The drawing under review shows one solid part. Ordinate dimensions are in mm from its lowest x, y, z. A direction names the side the tool comes from. Coordinates: 2 decimals unless noted, no trailing zeros. Order: outer loops, then holes, each group sorted by start corner. A loop starts at its lowest first (then second) coordinate and runs counter-clockwise, first axis right, second up. Notation, with made-up numbers: (-19.75, -35) -> (-1.75, -35) arc R22 cw to (-1.75, -26) -> close; hole circle Ø11 at (71, 2). An arc over 180 degrees is marked (long way). Use a Markdown table: item, result. Add a question column.
Q1. Add section A-A (x = 13.5). State the section outline as (y, z) points.
Q2. Machinability: for the marked faces 1 and 2, which of the approach directions +Z, -Z, +X, -X, +Y, -Y give a long, thin tool a straight path to every point of the face, cutting with its end or side? Answer none if there is none.
Q3. The part is to be moulded in two halves that separate along Y. For the marked faces 3, 4 and 5, say which applies: pulls with the +Y half, pulls with the -Y half, needs draft (parallel to the pull), parting line crosses it, or undercut.
Q4. Insertion check: pin 1 (0.9 mm diameter, centred on x = 9.5, z = 2.5, fed in from +Y); pin 2 (1.2 mm diameter, centred on y = 8, z = 1, fed in from +X); pin 3 (0.8 mm diameter, centred on y = 44.5, z = 1.5, fed in from +X). Each pin has a flat end and moves straight along its axis. Give the tip position at first contact, or say it passes through.
Q5. Add section B-B (y = 42.5). State the section outline as (x, z) points, then the cut area to 3 significant figures.
Q6. Add section C-C (x = 17). State the section outline as (y, z) points.
Q7. Wall thickness on probe 1 along Y at (x, z) = (11.5, 2); probe 2 along Y at (x, z) = (8.5, 0.7); probe 3 along Y at (x, z) = (14.25, 2.4): over which ranges is each line inside the solid? List them lowest first.
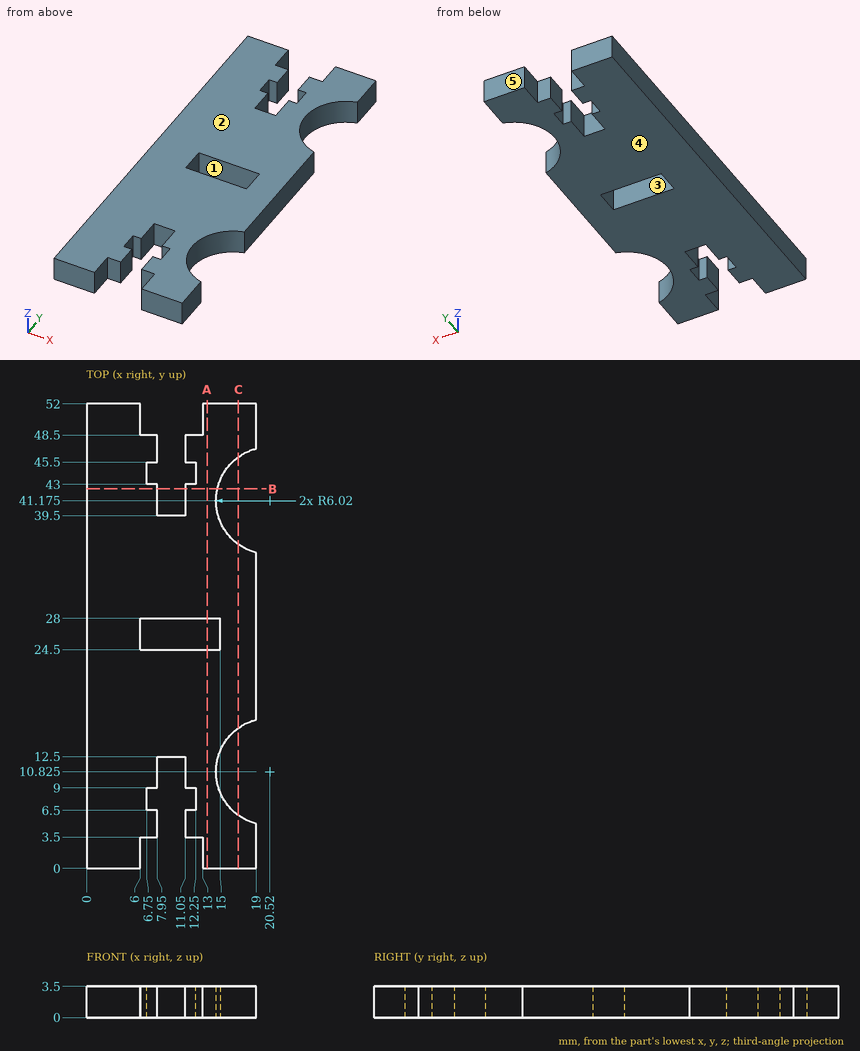
Established:
| question | item | result |
|---|---|---|
| 1 | outline | (0, 0) -> (24.5, 0) -> (24.5, 3.5) -> (0, 3.5) -> close; (28, 0) -> (52, 0) -> (52, 3.5) -> (28, 3.5) -> close |
| 2 | face 1 | +Z, -Z |
| 2 | face 2 | +Z, +X, -X, +Y, -Y |
| 3 | face 3 | undercut |
| 3 | face 4 | needs draft |
| 3 | face 5 | pulls with the +Y half |
| 4 | pin 1 | y = 39.5 |
| 4 | pin 2 | x = 15.57 |
| 4 | pin 3 | x = 15.79 |
| 5 | outline | (0, 0) -> (7.95, 0) -> (7.95, 3.5) -> (0, 3.5) -> close; (11.05, 0) -> (14.65, 0) -> (14.65, 3.5) -> (11.05, 3.5) -> close |
| 5 | area | 40.4 mm^2 |
| 6 | outline | (0, 0) -> (5.94, 0) -> (5.94, 3.5) -> (0, 3.5) -> close; (15.71, 0) -> (36.29, 0) -> (36.29, 3.5) -> (15.71, 3.5) -> close; (46.06, 0) -> (52, 0) -> (52, 3.5) -> (46.06, 3.5) -> close |
| 7 | probe 1 | 3.5 to 6.5, 9 to 24.5, 28 to 43, 45.5 to 48.5 |
| 7 | probe 2 | 12.5 to 24.5, 28 to 39.5 |
| 7 | probe 3 | 0 to 24.5, 28 to 52 |
